Geometry check sheet. Reference: the model listing, model coordinates, mm. Face numbers are marked on the shaded views. Give positions to 0.01 mm unless a question says otherwise; leave off trailing zeros. Write each loop counter-clockwise with the first axis right and the second up, starting at its lowest first coordinate (ties: lowest second). Pieces come first, ordered by that corner, then holes. Notation, with made-up numbers: (32.5, -21.75) - (75.5, -21.75) arc R22 ccw to (75.5, 12.25) - close; hole circle Ø5 at (66.5, 21). An arc over 180 degrees is marked (long way). Use a Markdown table: item, result.
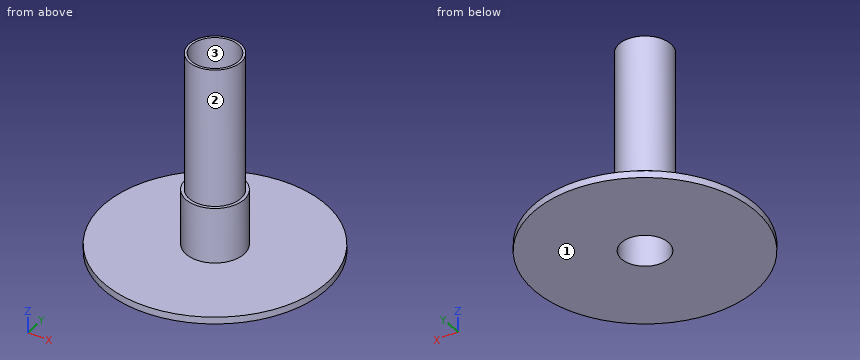
```python
from build123d import *

# Parameters (mm, degrees)
SKETCH019_R     = 80.456645
PAD008_DEPTH    = 5
SKETCH020_R     = 21
PAD009_DEPTH    = 40
SKETCH021_R     = 18.75
PAD010_DEPTH    = 100
SKETCH022_R     = 17
POCKET011_DEPTH = 145.001


with BuildPart() as part:
    # Sketch019 → Pad008 (new body)
    with BuildSketch(Plane.XY):
        Circle(SKETCH019_R)
    extrude(amount=PAD008_DEPTH)

    # Sketch020 (on Face3 of Pad008) → Pad009 (join)
    with BuildSketch(Plane.XY.offset(5)):
        Circle(SKETCH020_R)
    extrude(amount=PAD009_DEPTH)

    # Sketch021 (on Face5 of Pad009) → Pad010 (join)
    with BuildSketch(Plane.XY.offset(45)):
        Circle(SKETCH021_R)
    extrude(amount=PAD010_DEPTH)

    # Sketch022 (on Face7 of Pad010) → Pocket011 (cut, through all)
    with BuildSketch(Plane.XY.offset(145)):
        Circle(SKETCH022_R)
    extrude(amount=-POCKET011_DEPTH, mode=Mode.SUBTRACT)


solid = part.part
```
1) Section check A-A on x = 0. Record the boundary of the cut face in (y, z).
Working result:
| item | result |
|---|---|
| outline | (-80.46, 0) - (-17, 0) - (-17, 145) - (-18.75, 145) - (-18.75, 45) - (-21, 45) - (-21, 5) - (-80.46, 5) - close; (17, 0) - (80.46, 0) - (80.46, 5) - (21, 5) - (21, 45) - (18.75, 45) - (18.75, 145) - (17, 145) - close |
2) Section check C-C on z = 70. Record the boundary of the cut face in (x, y).
Working result:
| item | result |
|---|---|
| outline | circle Ø37.5 at (0, 0); hole circle Ø34 at (0, 0) |
3) Material ranges on L1, parallel to Y at x = 0, z = 98; L2, parallel to Z at x = -65.5, y = 45; L3, parallel to Y at x = -7, z = 8, recorded low to high. Write a range as from..to.
Working result:
| item | result |
|---|---|
| L1 | y = -18.75..-17, 17..18.75 |
| L2 | z = 0..5 |
| L3 | y = -19.8..-15.49, 15.49..19.8 |
4) Section check D-D on x = -24.5. Record the boundary of the cut face in (y, z).
Working result:
| item | result |
|---|---|
| outline | (-76.64, 0) - (76.64, 0) - (76.64, 5) - (-76.64, 5) - close |
5) Depth check by flat-ended pin: P1, Ø2, axis at y = -11, z = 83, coming from the -X side; P2, Ø2, axis at x = -6, z = 113.5, coming from the -Y side; P3, Ø4, axis at x = 64, y = -30.5, coming from the +Z side. Enter the tip coordinate at first touch or a pass-through.
Working result:
| item | result |
|---|---|
| P1 | stops at x = -15.86 |
| P2 | stops at y = -18.07 |
| P3 | stops at z = 5 |
6) Mould release check, pull along X, two halves, no side actions. Record for the marked faces 1, 2 and 3: pulls with the +X half, pulls with the -X half, needs draft (parallel to the pull), parting line crosses it, or undercut.
Working result:
| item | result |
|---|---|
| face 1 | needs draft |
| face 2 | parting line crosses it |
| face 3 | undercut |
